```python
from build123d import *

# Parameters (mm, degrees)
SKETCH1_W             = 203.2
SKETCH1_H             = 101.6
BOSS_EXTRUDE1_DEPTH   = 6.35
F_6_CLEARANCE_HOLE1_D = 3.7973


with BuildPart() as part:
    # Sketch1 → Boss-Extrude1 (new body)
    with BuildSketch(Plane.XY):
        with Locations((101.6, 50.8)):
            Rectangle(SKETCH1_W, SKETCH1_H)
    extrude(amount=BOSS_EXTRUDE1_DEPTH)

    # #6 Clearance Hole1 (through all)
    with Locations(Plane.XY.offset(6.35)):
        with Locations((3.175, 3.175), (3.175, 98.425), (200.025, 98.425), (200.025, 3.175), (101.6, 95.25), (101.6, 6.35)):
            Hole(F_6_CLEARANCE_HOLE1_D / 2)


solid = part.part
```
Here's how the part is built. I have some questions about the finished solid (model axes, mm). Give positions to 0.01 mm unless a question says otherwise; leave off trailing zeros. Loops run counter-clockwise (first coordinate to the right, second up) from the corner with the lowest first, then second, coordinate; pieces in that order, holes last. Notation, with made-up numbers: M 3.25,72.5 L 43.25,72.5 A32 cw 43.25,101.5 Z; hole C 33,-38.75 d4. An arc over 180 degrees is marked long. Put each result on its own line as item: value. Start each with the question number.
(1) I need wall thicknesses on line 1 along Y through (x, z) = (102.5, 4.5). Which ranges of the line are inside material? Lowest first, please. Write a range as [from, to].
(2) I want a section at A-A on x = 101.6. Please give me the cut outline in (y, z).
(3) If we mould it in two halves opening along X, with no side actions, what happens to faces 1 (the flat face through (100, 52, 0)), 2 (the cylindrical face through (100.724, 93.566, 3.131)), 3 (the flat face through (203.2, 50, 3)), 4 (the cylindrical face through (1.364, 3.745, 3.131))? For each: +X half, -X half, draft (parallel to the pull), parting line (faces both ways), or undercut.
Answer block:
1. line 1: [0, 4.68], [8.02, 93.58], [96.92, 101.6]
2. outline: M 0,0 L 4.45,0 L 4.45,6.35 L 0,6.35 Z; M 8.25,0 L 93.35,0 L 93.35,6.35 L 8.25,6.35 Z; M 97.15,0 L 101.6,0 L 101.6,6.35 L 97.15,6.35 Z
3. face 1: draft
3. face 2: undercut
3. face 3: +X half
3. face 4: undercut
